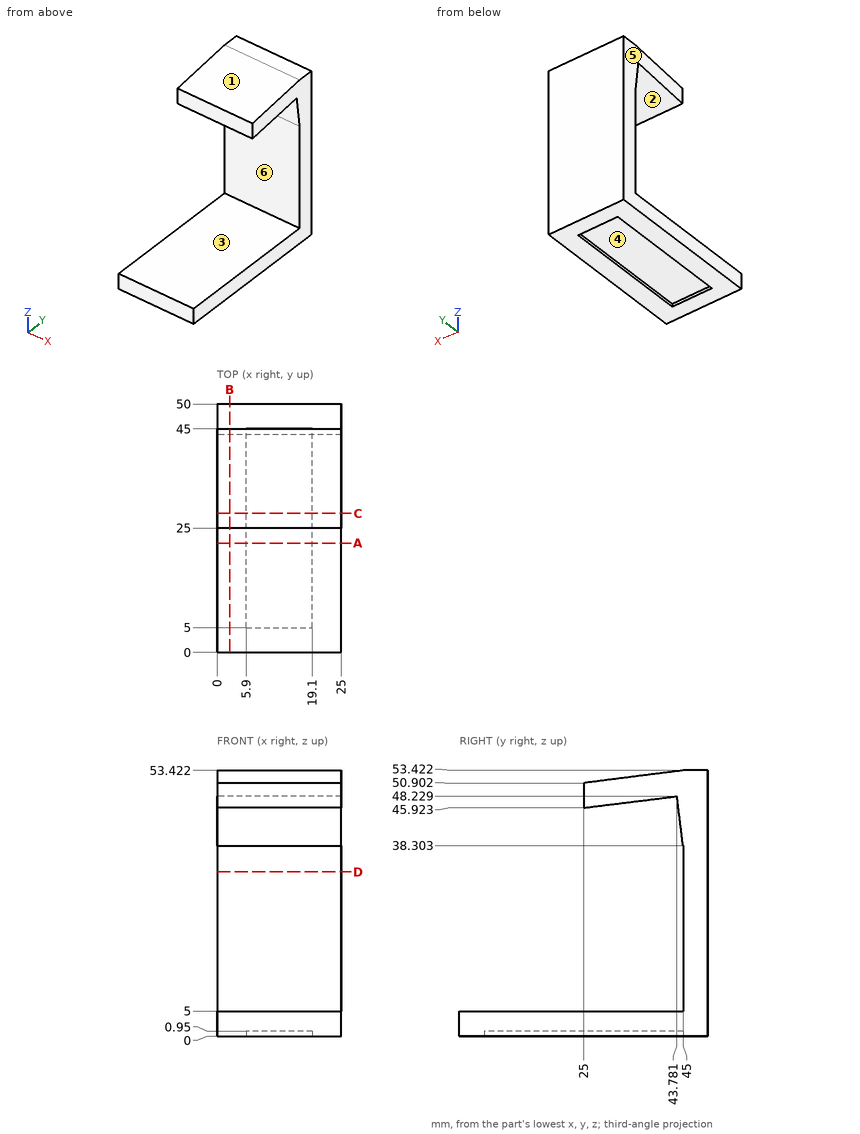
Check sheet for the drawn part. Datum: minimum x, y, z corner. Units: mm. A direction names the side the tool comes from. Round coordinates to 2 decimals unless told otherwise and drop trailing zeros. Order: outer loops, then holes, each group sorted by start corner. A loop starts at its lowest first (then second) coordinate and runs counter-clockwise, first axis right, second up. Notation, with made-up numbers: (47, -35) -> (71, -35) arc R21 cw to (71, -3) -> close; hole circle Ø1 at (-15.75, -10). An arc over 180 degrees is marked (long way). Put each result on its own line as item: value. Start each with the question number.
(1) Section check D-D (z = 33). Enter the section's corners in (x, y), then the cut area to 3 significant figures.
(2) Depth check by flat-ended pin: pin 1 Ø2 at (y, z) = (40, 45) entering from +X; pin 2 Ø3 at (x, y) = (20.5, 9.5) entering from +Z; pin 3 Ø6 at (x, z) = (3, 26.5) entering from -Y; pin 4 Ø1.5 at (x, y) = (14, 43) entering from -Z. Enter the tip coordinate at first touch or a pass-through.
(3) Material ranges on line 1 along Y through (x, z) = (15.25, 37); line 2 along Z through (x, y) = (7.5, 14.5); line 3 along Z through (x, y) = (4, 18.5), recorded low to high.
(4) Draft check along X on the marked faces 4, 5 and 6. Enter one of: +X half, -X half, draft (parallel to the pull), parting line (faces both ways), or undercut.
(5) Section check B-B (x = 2.5). Enter the section's corners in (y, z).
(6) Tool access check on the marked faces 1, 2 and 3. Record the directions out of +Z, -Z, +X, -X, +Y, -Y that give a thin tool (end or side, any length) a straight path to the whole face; none if there is none.
(7) Section check C-C (y = 28). Enter the section's corners in (x, z).
(8) Section check A-A (y = 22). Enter the section's corners in (x, z).
Completed:
1. outline: (0, 45) -> (25, 45) -> (25, 50) -> (0, 50) -> close
1. area: 125 mm2
2. pin 1: passes through
2. pin 2: stops at z = 5
2. pin 3: stops at y = 45
2. pin 4: stops at z = 0.95
3. line 1: y = 45 to 50
3. line 2: z = 0.95 to 5
3. line 3: z = 0 to 5
4. face 4: undercut
4. face 5: -X half
4. face 6: draft
5. outline: (0, 0) -> (50, 0) -> (50, 53.42) -> (45, 53.42) -> (25, 50.9) -> (25, 45.92) -> (43.78, 48.23) -> (45, 38.3) -> (45, 5) -> (0, 5) -> close
6. face 1: +Z, +X, -X, -Y
6. face 2: +X, -X
6. face 3: +X, -X, -Y
7. outline: (0, 0) -> (5.9, 0) -> (5.9, 0.95) -> (19.1, 0.95) -> (19.1, 0) -> (25, 0) -> (25, 5) -> (0, 5) -> close; (0, 46.29) -> (25, 46.29) -> (25, 51.28) -> (0, 51.28) -> close
8. outline: (0, 0) -> (5.9, 0) -> (5.9, 0.95) -> (19.1, 0.95) -> (19.1, 0) -> (25, 0) -> (25, 5) -> (0, 5) -> close
